Design review of the part built by this model. Coordinates are the model's own, in mm. Face numbers are marked on the shaded views. A direction names the side the tool comes from. Give positions to 0.01 mm unless a question says otherwise; leave off trailing zeros. Write each loop counter-clockwise with the first axis right and the second up, starting at its lowest first coordinate (ties: lowest second). Pieces come first, ordered by that corner, then holes. Notation, with made-up numbers: (24.25, 51) -> (34.25, 51) arc R35 cw to (34.25, 85) -> close; hole circle Ø6 at (-4, -34). An arc over 180 degrees is marked (long way). Answer as a JSON object with one key per item and string values.
```python
from build123d import *

# Parameters (mm, degrees)
F1_DEPTH     = 44.45
F4_DEPTH     = 98.5780825813
F5_SIZE      = 7.62
F6_T1_DEPTH  = 219.6945102582
F6_T3_DEPTH  = 31.6780747894
F6_T5_DEPTH  = 188.9400373947
F6_T7_DEPTH  = 31.6780747894
F6_T9_DEPTH  = 31.993119976
F6_T11_DEPTH = 19.558
F6_T13_DEPTH = 95.0320985588
F6_T19_DEPTH = 188.9400373947
F6_T23_DEPTH = 22.8240373947
F6_T30_DEPTH = 22.8240373947
F6_T34_DEPTH = 188.9400373947
F6_T41_DEPTH = 31.993119976
F6_T45_DEPTH = 188.9400373947
F7_T         = 3.81
F7_T3_DEPTH  = 9.8197045255
F7_T5_DEPTH  = 50.8
F7_T7_DEPTH  = 9.8197045256
F7_T9_DEPTH  = 9.8197045255
F8_R         = 4.0894
F8_R_2       = 1.8415
F9_DEPTH     = 40.64
F10_DEPTH    = 127


# Not quite as in the source:
# - a fillet or chamfer that OpenCascade refuses, or shapes differently, is made with other operations: its cross-section is extruded or revolved along the edge and cut away or added
# - a shell that OpenCascade refuses in one call is made with other operations: the cavity is built on its own and cut out


with BuildPart() as f1:
    # F0 (on Front) → F1 (new body)
    with BuildSketch(Plane.XZ):
        Polygon((-27.6737742102, 28.612719938), (-93.7137742102, 28.612719938), (-96.8887742102, -69.9643626433), (-17.5137742102, -69.9643626433), (12.7122257898, -69.9643626433), (12.7122257898, -41.237280062), (198.3862257898, -41.237280062), (198.3862257898, -16.091280062), (12.7122257898, -16.091280062), (12.7122257898, 3.466719938), (198.3862257898, 3.466719938), (198.3862257898, 28.612719938), align=None)
    extrude(amount=F1_DEPTH)

    # F2 (on face) → F4 (cut, through all)
    with BuildSketch(Plane(origin=(0, 0, -69.9643626433), x_dir=(1, 0, 0), z_dir=(0, 0, -1))):
        Polygon((-96.8887742102, 44.45), (-96.8887742102, 8.89), (-30.8487742102, 44.45), align=None)
    extrude(amount=-F4_DEPTH, mode=Mode.SUBTRACT)

    # F5
    f5_edges = [f1.edges().sort_by_distance(p)[0] for p in [
        (-62.281274, -27.524808, 28.61272),
    ]]
    chamfer(f5_edges, length=F5_SIZE)

    # F6: chamfer of 1.27 on 9 edges, made by hand

    # F6_s2 → F6_t1 (cut)
    with BuildSketch(Plane.YZ.offset(-18.0422470736)):
        Polygon((-43.18, 28.612719938), (-44.45, 27.342719938), (-44.45, 28.612719938), align=None)
    extrude(amount=F6_T1_DEPTH, mode=Mode.SUBTRACT)

    # F6_s4 → F6_t3 (cut)
    with BuildSketch(Plane.XY.offset(0.2006825433)):
        Polygon((197.1162257898, -44.45), (198.3862257898, -43.18), (198.3862257898, -44.45), align=None)
    extrude(amount=F6_T3_DEPTH, mode=Mode.SUBTRACT)

    # F6_s6 → F6_t5 (cut)
    with BuildSketch(Plane.YZ.offset(12.7122257898)):
        Polygon((-44.45, 4.736719938), (-43.18, 3.466719938), (-44.45, 3.466719938), align=None)
        Polygon((-44.45, -17.361280062), (-43.18, -16.091280062), (-44.45, -16.091280062), align=None)
        Polygon((-44.45, -39.967280062), (-43.18, -41.237280062), (-44.45, -41.237280062), align=None)
    extrude(amount=F6_T5_DEPTH, mode=Mode.SUBTRACT)

    # F6_s8 → F6_t7 (cut)
    with BuildSketch(Plane.XY.offset(-44.5033174567)):
        Polygon((197.1162257898, -44.45), (198.3862257898, -43.18), (198.3862257898, -44.45), align=None)
    extrude(amount=F6_T7_DEPTH, mode=Mode.SUBTRACT)

    # F6_s10 → F6_t9 (cut)
    with BuildSketch(Plane.XY.offset(-73.230400038)):
        Polygon((11.4422257898, -44.45), (12.7122257898, -43.18), (12.7122257898, -44.45), align=None)
    extrude(amount=F6_T9_DEPTH, mode=Mode.SUBTRACT)

    # F6_s12 → F6_t11 (cut)
    with BuildSketch(Plane.XY.offset(-16.091280062)):
        Polygon((11.4422257898, -44.45), (12.7122257898, -43.18), (12.7122257898, -44.45), align=None)
    extrude(amount=F6_T11_DEPTH, mode=Mode.SUBTRACT)

    # F6_s14 → F6_t13 (cut)
    with BuildSketch(Plane(origin=(-2.4104397516, 1.297929097, -74.8390924249), x_dir=(0.474099823, 0.8804710999, 0), z_dir=(0.0321867693, -0.0173313373, 0.9993315949))):
        Polygon((-53.0941334984, 78.8407390233), (-53.7623387855, 77.722372749), (-53.7623387855, 78.4811766705), align=None)
    extrude(amount=F6_T13_DEPTH, mode=Mode.SUBTRACT)


with BuildPart() as f6_tool17:
    # F6_s18 → F6_t19 (new body)
    with BuildSketch(Plane.YZ.offset(9.4461883951)):
        Polygon((-44.45, 4.736719938), (-43.18, 3.466719938), (-44.45, 3.466719938), align=None)
    extrude(amount=F6_T19_DEPTH)

    split(bisect_by=Plane.YZ.offset(12.7122257898), keep=Keep.BOTTOM)


with BuildPart() as f6_tool21:
    # F6_s22 → F6_t23 (new body)
    with BuildSketch(Plane.XY.offset(-16.091280062)):
        Polygon((11.4422257898, -44.45), (12.7122257898, -43.18), (12.7122257898, -44.45), align=None)
    extrude(amount=F6_T23_DEPTH)

    split(bisect_by=Plane.XY.offset(3.466719938), keep=Keep.TOP)


with BuildPart() as f6_tool17_1:
    add(f6_tool17.part)

    # F6_t25: intersect F6_tool21
    add(f6_tool21.part, mode=Mode.INTERSECT)


with BuildPart() as f1_1:
    add(f1.part)

    # F6_t15: cut F6_tool17
    add(f6_tool17_1.part, mode=Mode.SUBTRACT)


with BuildPart() as f6_tool28:
    # F6_s29 → F6_t30 (new body)
    with BuildSketch(Plane.XY.offset(-19.3573174567)):
        Polygon((11.4422257898, -44.45), (12.7122257898, -43.18), (12.7122257898, -44.45), align=None)
    extrude(amount=F6_T30_DEPTH)

    split(bisect_by=Plane.XY.offset(-16.091280062), keep=Keep.BOTTOM)


with BuildPart() as f6_tool32:
    # F6_s33 → F6_t34 (new body)
    with BuildSketch(Plane.YZ.offset(198.3862257898)):
        Polygon((-44.45, -17.361280062), (-43.18, -16.091280062), (-44.45, -16.091280062), align=None)
    extrude(amount=-F6_T34_DEPTH)

    split(bisect_by=Plane.YZ.offset(12.7122257898), keep=Keep.BOTTOM)


with BuildPart() as f6_tool28_1:
    add(f6_tool28.part)

    # F6_t36: intersect F6_tool32
    add(f6_tool32.part, mode=Mode.INTERSECT)


with BuildPart() as f1_2:
    add(f1_1.part)

    # F6_t26: cut F6_tool28
    add(f6_tool28_1.part, mode=Mode.SUBTRACT)


with BuildPart() as f6_tool39:
    # F6_s40 → F6_t41 (new body)
    with BuildSketch(Plane.XY.offset(-69.9643626433)):
        Polygon((11.4422257898, -44.45), (12.7122257898, -43.18), (12.7122257898, -44.45), align=None)
    extrude(amount=F6_T41_DEPTH)

    split(bisect_by=Plane.XY.offset(-41.237280062), keep=Keep.TOP)


with BuildPart() as f6_tool43:
    # F6_s44 → F6_t45 (new body)
    with BuildSketch(Plane.YZ.offset(9.4461883951)):
        Polygon((-44.45, -39.967280062), (-43.18, -41.237280062), (-44.45, -41.237280062), align=None)
    extrude(amount=F6_T45_DEPTH)

    split(bisect_by=Plane.YZ.offset(12.7122257898), keep=Keep.BOTTOM)


with BuildPart() as f6_tool39_1:
    add(f6_tool39.part)

    # F6_t47: intersect F6_tool43
    add(f6_tool43.part, mode=Mode.INTERSECT)


with BuildPart() as f1_3:
    add(f1_2.part)

    # F6_t37: cut F6_tool39
    add(f6_tool39_1.part, mode=Mode.SUBTRACT)

    # F7: shell of thickness 3.81, made by hand


with BuildPart() as f7_core1:
    # F7_t2: copy of F1
    add(f1_3.part)

    # the walls: a layer under each face that stays
    f7_faces = [f7_core1.faces().sort_by_distance(p)[0] for p in [
        (52.3362257898, -21.59, 28.612719938),
        (-95.3012742102, -4.8600664948, -20.6758213526),
        (-95.0796094442, -9.4847066882, -24.1721603779),
        (-63.5344983168, -26.8499947118, -24.4858213526),
        (83.1337257898, -44.45, -21.3108213526),
        (197.7512257898, -43.815, 16.039719938),
        (104.9142257898, -43.815, 4.101719938),
        (105.5492257898, -21.59, 3.466719938),
        (12.7122257898, -21.59, -6.312280062),
        (105.5492257898, -21.59, -16.091280062),
        (198.3862257898, -21.59, -28.664280062),
        (105.5492257898, -21.59, -41.237280062),
        (12.7122257898, -21.59, -55.6008213526),
        (12.0772257898, -43.815, -6.312280062),
        (104.9142257898, -43.815, -16.726280062),
        (197.7512257898, -43.815, -28.664280062),
        (104.9142257898, -43.815, -40.602280062),
        (12.0772257898, -43.815, -54.9658213526),
        (-42.0882742102, -22.225, -69.9643626433),
        (198.3862257898, -21.59, 16.039719938),
        (90.4656276778, -43.815, 27.977719938),
        (-57.0896392603, -25.9930745223, 24.802719938),
    ]]
    thicken(f7_faces, amount=-F7_T, mode=Mode.SUBTRACT)

    # F7_s4 → F7_t3 (cut)
    with BuildSketch(Plane(origin=(-9.1117935238, -9.1117935238, 9.1117935238), x_dir=(0.7071067812, -0.7071067812, 0), z_dir=(-0.5773502692, -0.5773502692, 0.5773502692))):
        Polygon((39.5789218716, -9.640847327), (37.6167718716, -6.3082949707), (35.7117718716, -7.4081472335), (35.7117718716, -9.6078517591), align=None)
    extrude(amount=F7_T3_DEPTH, mode=Mode.SUBTRACT)

    # F7_s6 → F7_t5 (cut)
    with BuildSketch(Plane.XZ.offset(-3.81)):
        Polygon((12.7503257898, 3.428619938), (12.7122257898, 7.276719938), (8.9022257898, 7.276719938), (8.9022257898, 3.466719938), align=None)
        Polygon((12.7503257898, -16.053180062), (8.9022257898, -16.091280062), (8.9022257898, -19.901280062), (12.7122257898, -19.901280062), align=None)
        Polygon((12.7503257898, -41.275380062), (12.7122257898, -37.427280062), (8.9022257898, -37.427280062), (8.9022257898, -41.237280062), align=None)
    extrude(amount=F7_T5_DEPTH, mode=Mode.SUBTRACT)

    # F7_s8 → F7_t7 (cut)
    with BuildSketch(Plane(origin=(-13.3199802318, -13.3199802318, -13.3199802318), x_dir=(0.7071067812, -0.7071067812, 0), z_dir=(-0.5773502692, -0.5773502692, -0.5773502692))):
        Polygon((39.5789218716, -0.6670628499), (35.7117718716, -0.7000584178), (35.7117718716, -2.8997629434), (37.6167718716, -3.9996152062), align=None)
    extrude(amount=F7_T7_DEPTH, mode=Mode.SUBTRACT)

    # F7_s10 → F7_t9 (cut)
    with BuildSketch(Plane(origin=(0.1201307583, 0.1201307583, -0.1201307583), x_dir=(-0.7071067812, 0.7071067812, 0), z_dir=(0.5773502692, 0.5773502692, -0.5773502692))):
        Polygon((-39.5789218716, -46.1415104808), (-37.6167718716, -42.8089581245), (-35.7117718716, -43.9088103873), (-35.7117718716, -46.1085149129), align=None)
    extrude(amount=F7_T9_DEPTH, mode=Mode.SUBTRACT)


with BuildPart() as f1_4:
    add(f1_3.part)

    # what is left inside the walls is the cavity
    f7_cavity = [f7_core1.part.solids().sort_by_distance(p)[0] for p in [
        (50.81107, -0.0381, -35.835335),
    ]]
    add(f7_cavity, mode=Mode.SUBTRACT)

    # F8 (on face) → F9 (join, through all)
    with BuildSketch(Plane(origin=(0, -40.64, 0), x_dir=(-1, 0, 0), z_dir=(0, 1, 0))):
        with Locations((-167.5252257898, 14.642719938)):
            Circle(F8_R)
        with Locations((-167.5252257898, 14.642719938)):
            Circle(F8_R_2, mode=Mode.SUBTRACT)
        with Locations((-109.7656257898, 14.642719938)):
            Circle(F8_R)
        with Locations((-109.7656257898, 14.642719938)):
            Circle(F8_R_2, mode=Mode.SUBTRACT)
        with Locations((9.3857742102, -44.920280062)):
            Circle(F8_R)
        with Locations((9.3857742102, -44.920280062)):
            Circle(F8_R_2, mode=Mode.SUBTRACT)
        with Locations((9.3857742102, 4.609719938)):
            Circle(F8_R)
        with Locations((9.3857742102, 4.609719938)):
            Circle(F8_R_2, mode=Mode.SUBTRACT)
    extrude(amount=F9_DEPTH)

    # F3 (on face) → F10 (cut, symmetric)
    with BuildSketch(Plane(origin=(0, 0, -41.237280062), x_dir=(1, 0, 0), z_dir=(0, 0, -1))):
        with BuildLine():
            Line((-70.9720987785, 3.4942372568), (-96.1306024302, 0))
            Line((-96.1306024302, 0), (198.3862257898, 0))
            Line((198.3862257898, 0), (198.3862257898, 24.13))
            ThreePointArc((198.3862257898, 24.13), (81.1301273633, 25.39290124), (-36.0551004282, 21.1255923438))
            Line((-36.0551004282, 21.1255923438), (-70.9720987785, 3.4942372568))
        make_face()
    extrude(amount=F10_DEPTH, both=True, mode=Mode.SUBTRACT)


solid = f1_4.part
```
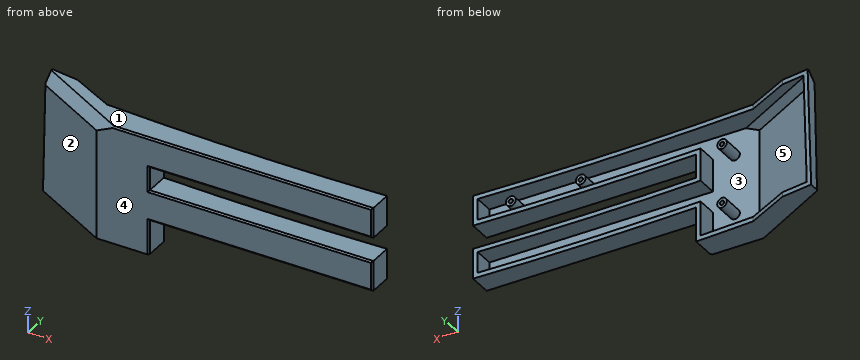
(1) We need section D-D, the plane y = -18. State the section outline as (x, z) points (3 decimals), then the cut area to 3 significant figures.
Here are the results:
{"outline": "(-79.97, -69.964) -> (-42.245, -69.964) -> (-42.245, -66.154) -> (-71.934, -66.154) -> (-71.934, 19.415) -> (-60.569, 24.803) -> (-42.245, 24.803) -> (-42.245, 28.613) -> (-63.898, 28.613) -> (-79.97, 20.993) -> close", "area": "988 mm²"}
(2) We need section A-A, the plane y = -32.5. Give the number of separate pieces and of enclosed holes in the cut face, then the cut area to 3 significant figures.
Here are the results:
{"separate pieces": "5", "enclosed holes": "5", "area": "4,550 mm²"}
(3) Clearance check with flat-ended pins moving along their axes: pin 1 (3 mm diameter, centred on x = 23.5, y = -36, fed in from -Z); pin 2 (1 mm diameter, centred on x = 80.5, z = -14.5, fed in from +Y); pin 3 (1 mm diameter, centred on x = -50.5, y = -33, fed in from +Z); pin 4 (1.8 mm diameter, centred on x = -10, z = -45, fed in from +Y). State where each tip first meets the part, or that it passes through.
Here are the results:
{"pin 1": "stops at z = -41.24", "pin 2": "passes through", "pin 3": "stops at z = 22.26", "pin 4": "stops at y = -40.64"}
(4) For the marked faces 4 and 5, list the 3-axis set-ups (+Z, -Z, +X, -X, +Y, -Y) from which the entire face can be reached by the end or side of a thin tool; tool diameter is ignored.
Here are the results:
{"face 4": "+Z, -Z, +X, -X, -Y", "face 5": "+Y"}
(5) For line 1 along Z through (x, y) = (91, -32); line 2 along Z through (x, y) = (169, -30.5); line 3 along Y through (x, z) = (-17, 24), list the stretches that pass through material, from the lowest coordinate up.
Here are the results:
{"line 1": "z = -41.24 to -37.43, -19.9 to -16.09, 3.47 to 7.28, 24.8 to 28.61", "line 2": "z = -41.24 to -37.43, -19.9 to -16.09, 3.47 to 7.28, 10.83 to 13.54, 15.75 to 18.46, 24.8 to 28.61", "line 3": "y = -44.45 to -40.64"}
(6) We need section C-C, the plane z = -10. State the section outline as (x, y) points, then the cut area to 3 significant figures.
Here are the results:
{"outline": "(-94.96, -9.17) -> (-94.29, -10.29) -> (-30.85, -44.45) -> (11.44, -44.45) -> (12.71, -43.18) -> (12.71, -23.57) arc R2486.25 cw to (8.9, -23.42) -> (8.9, -40.64) -> (-29.89, -40.64) -> (-91.15, -7.66) -> (-91.15, -0.69) -> (-94.96, -0.16) -> close", "area": "532 mm²"}
(7) The part is to be moulded in two halves that separate along X. For the marked faces 1, 2 and 3, say which applies: +X half, -X half, draft (parallel to the pull), parting line (faces both ways), or undercut.
Here are the results:
{"face 1": "draft", "face 2": "-X half", "face 3": "undercut"}
(8) We need section B-B, the plane x = 55. State the section outline as (y, z) points.
Here are the results:
{"outline": "(-44.45, -39.97) -> (-43.18, -41.24) -> (-24.92, -41.24) -> (-24.92, -37.43) -> (-40.64, -37.43) -> (-40.64, -19.9) -> (-24.92, -19.9) -> (-24.92, -16.09) -> (-43.18, -16.09) -> (-44.45, -17.36) -> close; (-44.45, 4.74) -> (-43.18, 3.47) -> (-24.92, 3.47) -> (-24.92, 7.28) -> (-40.64, 7.28) -> (-40.64, 24.8) -> (-24.92, 24.8) -> (-24.92, 28.61) -> (-43.18, 28.61) -> (-44.45, 27.34) -> close"}
